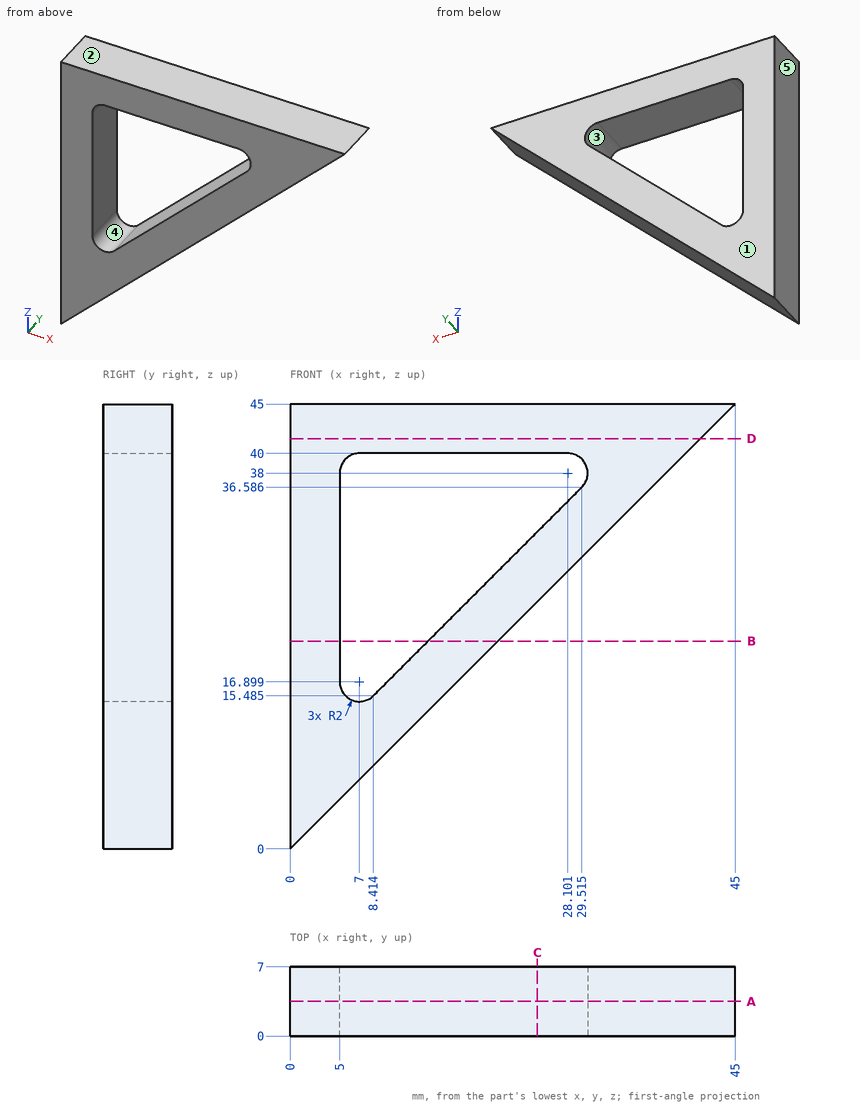
Design review of the part shown in the three views and the two pictorial views. Dimensions are in mm from the part's minimum x, y and z. A direction names the side the tool comes from. Give positions to 0.01 mm unless a question says otherwise; leave off trailing zeros. Order: outer loops, then holes, each group sorted by start corner. A loop starts at its lowest first (then second) coordinate and runs counter-clockwise, first axis right, second up. Notation, with made-up numbers: M 20.5,-38 L 45.5,-38 A22 cw 45.5,-20 Z; hole C -37,24.5 d1. An arc over 180 degrees is marked long. Answer in a Markdown table with one row per item. Add a question column.
(1) Consider section D-D on z = 41.5. State the section outline as (x, y) points.
(2) Consider section C-C on x = 25. State the section outline as (y, z) points.
(3) Consider section B-B on z = 21. State the section outline as (x, y) points.
(4) For the marked faces 4 and 5, list the 3-axis set-ups (+Z, -Z, +X, -X, +Y, -Y) from which the entire face can be reached by the end or side of a thin tool; tool diameter is ignored.
(5) For pin 1 (1 mm diameter, centred on x = 33, y = 2, fed in from -Z); pin 2 (1 mm diameter, centred on x = 32.5, y = 5, fed in from -Z); pin 3 (1.5 mm diameter, centred on y = 3, z = 40.5, fed in from -X); pin 4 (1 mm diameter, centred on x = 10.5, y = 1.5, fed in from -Z), all flat-tipped, find the tip position at first contact; note any pin that passes through.
(6) Mouldability with a two-part tool opening along Z and no side actions: class the marked faces 1, 2 and 3 as +Z half, -Z half, draft (parallel to the pull), parting line (faces both ways), or undercut.
(7) Wall thickness on probe 1 along X at (y, z) = (6.75, 38); probe 2 along X at (y, z) = (1.75, 17); probe 3 along Z at (x, y) = (6, 1.25) (1 decimal): over which ranges is each line inside the solid? List them lowest first. Write a range as [from, to].
(8) Consider section A-A on y = 3.5. State the section outline as (x, z) points (1 decimal).
Evaluation:
| question | item | result |
|---|---|---|
| 1 | outline | M 0,0 L 41.5,0 L 41.5,7 L 0,7 Z |
| 2 | outline | M 0,25 L 7,25 L 7,32.07 L 0,32.07 Z; M 0,40 L 7,40 L 7,45 L 0,45 Z |
| 3 | outline | M 0,0 L 5,0 L 5,7 L 0,7 Z; M 13.93,0 L 21,0 L 21,7 L 13.93,7 Z |
| 4 | face 4 | +Y, -Y |
| 4 | face 5 | +Z, -Z, -X, +Y, -Y |
| 5 | pin 1 | stops at z = 32.5 |
| 5 | pin 2 | stops at z = 32 |
| 5 | pin 3 | stops at x = 0 |
| 5 | pin 4 | stops at z = 10 |
| 6 | face 1 | draft |
| 6 | face 2 | +Z half |
| 6 | face 3 | undercut |
| 7 | probe 1 | x = [0, 5], [30.1, 38] |
| 7 | probe 2 | x = [0, 5], [9.93, 17] |
| 7 | probe 3 | z = [6, 15.2], [39.7, 45] |
| 8 | outline | M 0,0 L 45,45 L 0,45 Z; hole M 5,16.9 A2 ccw 8.4,15.5 L 29.5,36.6 A2 ccw 28.1,40 L 7,40 A2 ccw 5,38 Z |
